Part print with two shaded views. Sizes in mm from the minimum x, y, z corner. Give positions to 0.01 mm unless a question says otherwise; leave off trailing zeros. Loops run counter-clockwise (first coordinate to the right, second up) from the corner with the lowest first, then second, coordinate; pieces in that order, holes last. Notation, with made-up numbers: M -19.75,-33.75 L 9.25,-33.75 A11 cw 9.25,-22.75 Z; hole C 33.5,58.25 d8. An arc over 180 degrees is marked long. Answer as a JSON object with one key per item and string values. Group by question number.
1. Slice it at A-A (z = 360). List the corners of the cut face in (x, y).
2. Drill centre lines: line 1 along X through (y, z) = (201, 351.5); line 2 along Z through (x, y) = (365, 286.5); line 3 along Z through (x, y) = (360, 273). Where is each one in solid material? Low to high. Write a range as [from, to].
3. Mould opens along Z. For the marked faces 1, 2 and 3 say: released by +Z, released by -Z, zero draft, split by the parting line, or undercut.
4. Slice it at C-C (y = 192.5). List the corners of the cut face in (x, z), then the cut area to 3 significant figures.
5. Drop flat-ended pins along their axis: pin 1 Ø3 at (x, y) = (78, 264.5) entering from -Z; pin 2 Ø10 at (x, y) = (198.5, 284.5) entering from -Z; pin 3 Ø6 at (y, z) = (165.5, 127) entering from -X. Give the stop position or say it passes through.
6. Slice it at B-B (x = 360). List the corners of the cut face in (y, z), then the cut area to 3 significant figures.
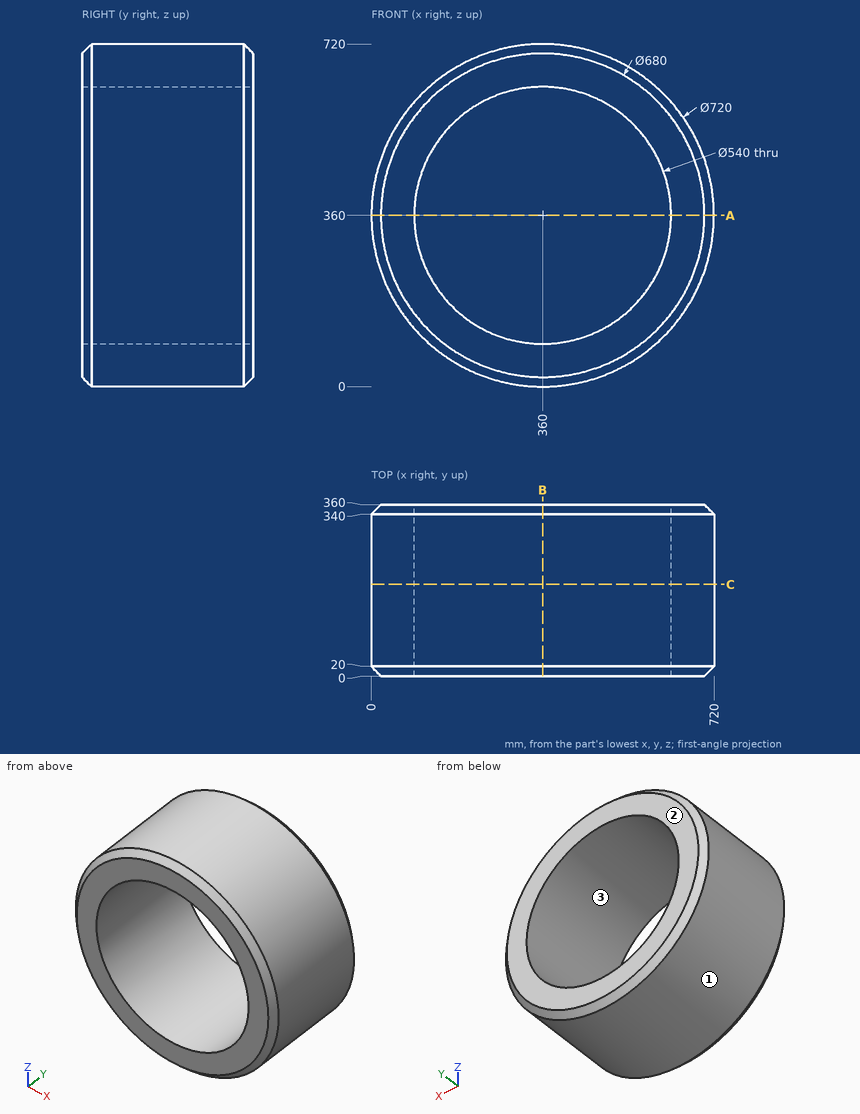
Established:
{
 "1": {"outline": "M 0,20 L 20,0 L 90,0 L 90,360 L 20,360 L 0,340 Z; M 630,0 L 700,0 L 720,20 L 720,340 L 700,360 L 630,360 Z"},
 "2": {"line 1": "x = [0.1, 90.13], [629.87, 719.9]", "line 2": "z = [0.03, 90.05], [629.95, 719.97]", "line 3": "z = [0, 90], [630, 720]"},
 "3": {"face 1": "split by the parting line", "face 2": "zero draft", "face 3": "undercut"},
 "4": {"outline": "C 360,360 d720; hole C 360,360 d540", "area": "178,000 mm^2"},
 "5": {"pin 1": "stops at z = 134.35", "pin 2": "stops at z = 35.8", "pin 3": "stops at x = 83.05"},
 "6": {"outline": "M 0,20 L 20,0 L 340,0 L 360,20 L 360,90 L 0,90 Z; M 0,630 L 360,630 L 360,700 L 340,720 L 20,720 L 0,700 Z", "area": "64,000 mm^2"}
}
